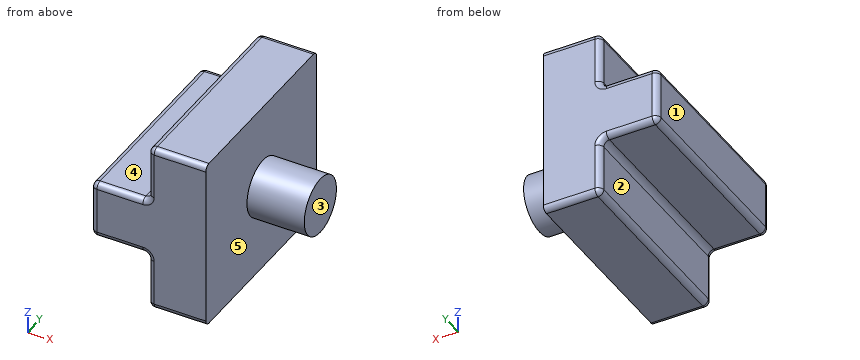
Autodesk Inventor part; units mm, degrees
ref_plane "YZ Plane" through (0, 0, 0) normal (1, 0, 0) x (0, 1, 0)
ref_plane "XZ Plane" through (0, 0, 0) normal (0, 1, 0) x (-1, 0, 0)
ref_plane "XY Plane" through (0, 0, 0) normal (0, 0, 1) x (1, 0, 0)
sketch "Sketch1" plane through (0, 0, 0) normal (0, 1, 0) x (-1, 0, 0)
  line L0 (0, 15.24) -> (0, -15.24)
  line L1 (0, -15.24) -> (10.16, -15.24)
  line L2 (10.16, -15.24) -> (10.16, -5.08)
  line L3 (10.16, -5.08) -> (20.32, -5.08)
  line L4 (20.32, -5.08) -> (20.32, 5.08)
  line L5 (20.32, 5.08) -> (10.16, 5.08)
  line L6 (10.16, 5.08) -> (10.16, 15.24)
  line L7 (10.16, 15.24) -> (0, 15.24)
  point P0 (0, 0)
  dimension "d1" = 10.16
  dimension "d2" = 10.16
  dimension "d3" = 10.16
  dimension "d4" = 15.24
  dimension "d5" = 10.16
extrude "Extrusion1" add sketch "Sketch1" along normal blind 35.052
sketch "Sketch2" plane through (0, 0, 15.24) normal (1, 0, 0) x (0, 0, -1)
  circle A0 centre (15.24, 18.1015) radius 5.08
  point P0 (15.24, 0)
  dimension "d8" = 10.16
extrude "Extrusion2" add sketch "Sketch2" along normal blind 10.16
fillet "Fillet1" radius 1.016 6 edges at (-10.16, 17.526, 5.08) (-10.16, 17.526, -5.08) (-20.32, 17.526, 5.08) (-20.32, 17.526, -5.08) (-10.16, 17.526, 15.24) (-10.16, 17.526, -15.24)
fillet "Fillet2" radius 1.016 26 edges at (-9.8624, 35.052, 14.9424) (-4.572, 35.052, 15.24) (-10.4576, 35.052, 5.3776) (-15.24, 35.052, 5.08) (-20.0224, 35.052, 4.7824) (-20.32, 35.052, 0) (-20.0224, 35.052, -4.7824) (-15.24, 35.052, -5.08) (-10.4576, 35.052, -5.3776) (-10.16, 35.052, -10.16) (-9.8624, 35.052, -14.9424) (-4.572, 35.052, -15.24) (-10.16, 35.052, 10.16) (-9.8624, 0, 14.9424) (-10.16, 0, 10.16) (-10.4576, 0, 5.3776) (-15.24, 0, 5.08) (-20.0224, 0, 4.7824) (-20.32, 0, 0) (-20.0224, 0, -4.7824) (-15.24, 0, -5.08) (-10.4576, 0, -5.3776) (-10.16, 0, -10.16) (-9.8624, 0, -14.9424) (-4.572, 0, -15.24) (-4.572, 0, 15.24)
properties part number "Slider2"
For this review, take the finished solid that the model builds, in its own axes (mm). Face numbers are marked on the shaded views. A direction names the side the tool comes from. Coordinates: 2 decimals unless noted, no trailing zeros. Loops run counter-clockwise (first coordinate to the right, second up) from the corner with the lowest first, then second, coordinate; pieces in that order, holes last. Notation, with made-up numbers: (-9, 81.25) - (22, 81.25) arc R19 cw to (22, 106.25) - close; hole circle Ø6 at (3.5, 54). An arc over 180 degrees is marked (long way). Use a Markdown table: item, result. Add a question column.
Item 1: We need section A-A (z = 0). Give the boundary of the cut face in (x, y).
Item 2: We need section C-C (y = 6.5). Give the boundary of the cut face in (x, z).
Item 3: Tool access review of the marked faces 1, 2, 3, 4 and 5: name each direction out of +Z, -Z, +X, -X, +Y, -Y from which nothing blocks a thin tool from reaching the whole face with its end or side.
Item 4: We need section B-B (x = -16). Give the boundary of the cut face in (y, z), and give its area (3 significant figures).
Item 5: For line 1 (X direction, y = 7.5, z = 14); line 2 (X direction, y = 24.5, z = -2); line 3 (Z direction, x = -14.5, y = 23.5), list the stretches that pass through material, from the lowest coordinate up.
Item 6: Insertion check: pin 1 Ø4 at (x, y) = (-16, 30.5) entering from -Z; pin 2 Ø6 at (y, z) = (20, 11.5) entering from -X; pin 3 Ø12 at (y, z) = (4, 1) entering from +X; pin 4 Ø3 at (x, z) = (-12, -8.5) entering from -Y. Each pin has a flat end and moves straight along its axis. Give the tip position at first contact, or say it passes through.
Item 7: We need section D-D (z = 8). Give the boundary of the cut face in (x, y), and give its area (3 significant figures).
Results list:
| question | item | result |
|---|---|---|
| 1 | outline | (-20.32, 1.02) arc R1.02 ccw to (-19.3, 0) - (0, 0) - (0, 13.02) - (10.16, 13.02) - (10.16, 23.18) - (0, 23.18) - (0, 35.05) - (-19.3, 35.05) arc R1.02 ccw to (-20.32, 34.04) - close |
| 2 | outline | (-20.32, -4.06) arc R1.02 ccw to (-19.3, -5.08) - (-11.18, -5.08) arc R1.02 cw to (-10.16, -6.1) - (-10.16, -14.22) arc R1.02 ccw to (-9.14, -15.24) - (0, -15.24) - (0, 15.24) - (-9.14, 15.24) arc R1.02 ccw to (-10.16, 14.22) - (-10.16, 6.1) arc R1.02 cw to (-11.18, 5.08) - (-19.3, 5.08) arc R1.02 ccw to (-20.32, 4.06) - close |
| 3 | face 1 | +Z, -Z, -X, +Y, -Y |
| 3 | face 2 | -Z, -X, +Y, -Y |
| 3 | face 3 | +Z, -Z, +X, +Y, -Y |
| 3 | face 4 | +Z, -X, +Y, -Y |
| 3 | face 5 | +X |
| 4 | outline | (0, -4.06) arc R1.02 ccw to (1.02, -5.08) - (34.04, -5.08) arc R1.02 ccw to (35.05, -4.06) - (35.05, 4.06) arc R1.02 ccw to (34.04, 5.08) - (1.02, 5.08) arc R1.02 ccw to (0, 4.06) - close |
| 4 | area | 355 mm^2 |
| 5 | line 1 | x = -10.16 to 0 |
| 5 | line 2 | x = -20.32 to 0 |
| 5 | line 3 | z = -5.08 to 5.08 |
| 6 | pin 1 | stops at z = -5.08 |
| 6 | pin 2 | stops at x = -10.16 |
| 6 | pin 3 | stops at x = 0 |
| 6 | pin 4 | passes through |
| 7 | outline | (-10.16, 1.02) arc R1.02 ccw to (-9.14, 0) - (0, 0) - (0, 35.05) - (-9.14, 35.05) arc R1.02 ccw to (-10.16, 34.04) - close |
| 7 | area | 356 mm^2 |
